```python
from build123d import *

# Parameters (mm, degrees)
PAD_DEPTH            = 1.2
CHAMFER_SIZE         = 0.6
BODY_PLACEMENT_ANGLE = 25


with BuildPart() as part:
    # Sketch027 → Pad (new body)
    with BuildSketch(Plane.XZ):
        with BuildLine():
            ThreePointArc((-5.306735, -5.013468), (0, -19), (5.306735, -5.013468))
            ThreePointArc((3.482545, -0.349116), (3.832911, -2.90098), (5.306735, -5.013468))
            ThreePointArc((3.482545, -0.349116), (0, 3.5), (-3.482545, -0.349116))
            ThreePointArc((-5.306735, -5.013468), (-3.832911, -2.90098), (-3.482545, -0.349116))
        make_face()
    extrude(amount=PAD_DEPTH)

    # Sketch030 → Groove (revolve, cut)
    with BuildSketch(Plane.YZ):
        Polygon((0, 2.75), (-0.6, 2.15), (-1.2, 2.15), (-1.2, 0), (0, 0), align=None)
    revolve(axis=Axis((0, 0, 0), (0, 1, 0)), mode=Mode.SUBTRACT)

    # Chamfer
    chamfer_edges = [part.edges().sort_by_distance(p)[0] for p in [
        (0, 0, -19),
    ]]
    chamfer(chamfer_edges, length=CHAMFER_SIZE)


with BuildPart() as part_1:
    # Body placement: moved
    add(part.part.moved(Location((-16, 98.75, 37.54))).rotate(Axis((-16, 98.75, 37.54), (1, 0, 0)), BODY_PLACEMENT_ANGLE))


solid = part_1.part
```
Geometry check sheet. Reference: the model listing, model coordinates, mm. Give positions to 0.01 mm unless a question says otherwise; leave off trailing zeros.
1) Material ranges on L1, parallel to Y at x = -11.5, z = 28.5; L2, parallel to Y at x = -14, z = 31.5; L3, parallel to Z at x = -22.5, y = 103.5, recorded low to high.
2) Gauge pin test, flat ends, axial feed: pin 1 (5 mm diameter, centred on x = -18, z = 31, fed in from -Y); pin 2 (1.5 mm diameter, centred on x = -18.5, z = 28.5, fed in from +Y); pin 3 (5 mm diameter, centred on x = -14.5, z = 37, fed in from +Y); pin 4 (1 mm diameter, centred on y = 100, z = 37.5, fed in from +X). Record the tip position at first contact, or that the pin passes through.
3) Release check for a two-part mould opening along X. For faces 1 (the flat face through (-16.112, 101.928, 27.886)), 2 (the cylindrical face through (-18.1, 98.13, 36.74)) record: pulls with the +X half, pulls with the -X half, needs draft (parallel to the pull), parting line crosses it, or undercut.
Computed:
1. L1: y = 101.64 to 102.97
1. L2: y = 100.24 to 101.57
1. L3: z = 24.51 to 27.35
2. pin 1: stops at y = 99.31
2. pin 2: stops at y = 103.32
2. pin 3: stops at y = 100.17
2. pin 4: passes through
3. face 1: needs draft
3. face 2: undercut
